from build123d import *

# Parameters (mm, degrees)
SALIENTE_EXTRUIR1_DEPTH = 3
CROQUIS2_R              = 2
SALIENTE_EXTRUIR2_DEPTH = 3
CROQUIS3_R              = 2
CORTAR_EXTRUIR1_DEPTH   = 108.087875812


with BuildPart() as part:
    # Croquis1 → Saliente-Extruir1 (new body)
    with BuildSketch(Plane(origin=(0, 0, 0), x_dir=(1, 0, 0), z_dir=(0, 1, 0))):
        Polygon((-22.435530086, -36.676217765), (-52.435530086, -36.676217765), (-52.435530086, 93.323782235), (47.564469914, 93.323782235), (47.564469914, 53.323782235), (-22.435530086, 53.323782235), align=None)
    extrude(amount=SALIENTE_EXTRUIR1_DEPTH)

    # Croquis2 → Saliente-Extruir2 (add, through all)
    with BuildSketch(Plane(origin=(0, 3, 0), x_dir=(1, 0, 0), z_dir=(0, 1, 0))):
        with Locations((37.564469914, 73.323782235)):
            Circle(CROQUIS2_R)
        with Locations((-35.435530086, 75.002673531)):
            Circle(CROQUIS2_R)
        with Locations((-37.435530086, 45.002673531)):
            Circle(CROQUIS2_R)
        with Locations((-37.435530086, -4.997326469)):
            Circle(CROQUIS2_R)
    extrude(amount=-SALIENTE_EXTRUIR2_DEPTH)

    # Croquis3 → Cortar-Extruir1 (cut, through all)
    with BuildSketch(Plane(origin=(0, 3, 0), x_dir=(1, 0, 0), z_dir=(0, 1, 0))):
        with Locations(Location((37.564469914, 73.323782235, 0), (0, 0, 270))):
            Circle(CROQUIS3_R)
        with Locations(Location((-37.435530086, 45.002673531, 0), (0, 0, 270))):
            Circle(CROQUIS3_R)
        with Locations(Location((-37.435530086, -4.997326469, 0), (0, 0, 270))):
            Circle(CROQUIS3_R)
        with Locations(Location((-35.435530086, 75.002673531, 0), (0, 0, 270))):
            Circle(CROQUIS3_R)
    extrude(amount=-CORTAR_EXTRUIR1_DEPTH, mode=Mode.SUBTRACT)


solid = part.part
Model file for the job. Use its own axes, mm. A direction names the side the tool comes from. Round coordinates to 2 decimals unless told otherwise and drop trailing zeros. Order: outer loops, then holes, each group sorted by start corner. A loop starts at its lowest first (then second) coordinate and runs counter-clockwise, first axis right, second up.
(1) 3-axis set-ups, long thin cutter, end or side, ignore diameter. For faces 5 (the face through (47.564, 1, -74)), 6 (the face through (-22.436, 1, -9)): which of +Z, -Z, +X, -X, +Y, -Y reach the whole face in a straight line?
(2) Band-saw the part on A-A (y = 2.1). List the corners of the cut face in (x, z).
(3) Band-saw the part on C-C (z = -31). List the corners of the cut face in (x, y), then the cut area to 3 significant figures.
(4) Band-saw the part on B-B (x = 11). List the corners of the cut face in (y, z), then the cut area to 3 significant figures.
(5) Drill centre lines: line 1 (Z direction, x = -36.5, y = 0.9); line 2 (Z direction, x = 9.5, y = 0.3); line 3 (X direction, y = 2.5, z = -27). Where is each one in solid material? Low to high.
(6) Pull direction Z, two halves, no side cores. Call faces 1 (the face through (-52.436, 1, -27)), 2 (the face through (-3, 1, -93.324)), 3 (the face through (13, 1, -53.324)), 4 (the face through (-36.835, 1.521, -43.095)): released by +Z, released by -Z, zero draft, split by the parting line, or undercut.
(7) Pin check, flat tip, straight feed: pin 1 (3 mm diameter, centred on x = -37.44, z = -45, fed in from -Y). Stop position of the tip, or through.
Verdict:
1. face 5: +Z, -Z, +X, +Y, -Y
1. face 6: +Z, +X, +Y, -Y
2. outline: (-52.44, -93.32) - (47.56, -93.32) - (47.56, -53.32) - (-22.44, -53.32) - (-22.44, 36.68) - (-52.44, 36.68) - close; hole circle Ø4 at (-37.44, -45); hole circle Ø4 at (-37.44, 5); hole circle Ø4 at (-35.44, -75); hole circle Ø4 at (37.56, -73.32)
3. outline: (-52.44, 0) - (-22.44, 0) - (-22.44, 3) - (-52.44, 3) - close
3. area: 90.0 mm2
4. outline: (0, -93.32) - (3, -93.32) - (3, -53.32) - (0, -53.32) - close
4. area: 120 mm2
5. line 1: z = -93.32 to -76.7, -73.31 to -46.77, -43.23 to 3.23, 6.77 to 36.68
5. line 2: z = -93.32 to -53.32
5. line 3: x = -52.44 to -22.44
6. face 1: zero draft
6. face 2: released by -Z
6. face 3: released by +Z
6. face 4: undercut
7. pin 1: passes through
